Read the model definition and answer for the solid it produces. Units are mm, in the model's axes. Face numbers are marked on the shaded views. A direction names the side the tool comes from. Round coordinates to 2 decimals unless told otherwise and drop trailing zeros. Order: outer loops, then holes, each group sorted by start corner. A loop starts at its lowest first (then second) coordinate and runs counter-clockwise, first axis right, second up. Notation, with made-up numbers: (86, 55) - (139, 55) arc R32 cw to (139, 88) - close; hole circle Ø2 at (-25.75, 53.5). An arc over 180 degrees is marked (long way). Answer as a JSON object with one key per item and string values. Group by question number.
Q1. Consider line 1 (Y direction, x = -30, z = 10.75); line 2 (Y direction, x = -13, z = 13); line 3 (X direction, y = -4.5, z = 13.75). Determine where each line is inside the solid, lowest interval first.
Q2. A cutting plane is placed at C-C on y = -7. Determine the outline of the cut face in (x, z).
Q3. A cutting plane is placed at D-D on x = -17.5. Determine the outline of the cut face in (y, z).
Q4. A tool of negligible diameter and unlimited length cuts with its end or side. For the marked faces 1 and 2, from which of +Z, -Z, +X, -X, +Y, -Y can it reach the whole face along a straight path? Write none if from no direction.
Q5. Given pin 1 Ø2.5 at (x, y) = (-30, 0) entering from +Z; pin 2 Ø3 at (y, z) = (-4, 11) entering from +X, each flat-ended and moving along its own axis, determine where each tip first touches the part or whether it passes through.
Q6. A cutting plane is placed at A-A on x = -30. Determine the outline of the cut face in (y, z).
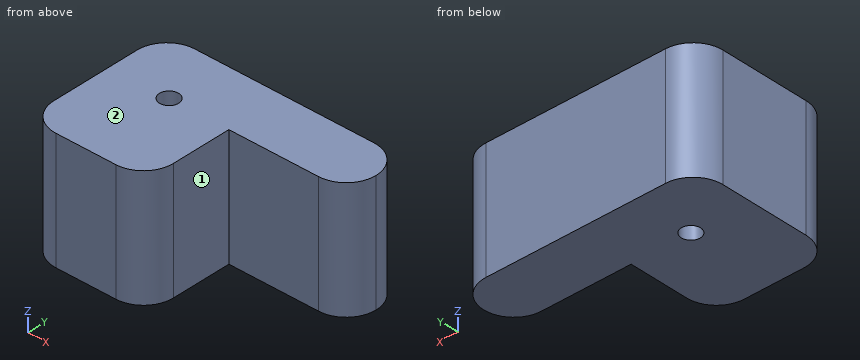
```python
from build123d import *

# Parameters (mm, degrees)
SKETCH_1_W          = 40
SKETCH_1_H          = 10
EXTRUDE_1_DEPTH     = 20
SKETCH_2_W          = 20
SKETCH_2_H          = 25
EXTRUDE_2_DEPTH     = 20
FILLET_1_R          = 5
SKETCH_3_R          = 1.6
CUT_EXTRUDE_1_DEPTH = 48.16990566


with BuildPart() as part:
    # 草图1 → 凸台-拉伸1 (new body)
    with BuildSketch(Plane.XY):
        with Locations((-20, 5)):
            Rectangle(SKETCH_1_W, SKETCH_1_H)
    extrude(amount=EXTRUDE_1_DEPTH)

    # 草图2 → 凸台-拉伸2 (add)
    with BuildSketch(Plane.XY.offset(20)):
        with Locations((-30, -2.5)):
            Rectangle(SKETCH_2_W, SKETCH_2_H)
    extrude(amount=-EXTRUDE_2_DEPTH)

    # 圆角1
    fillet_1_edges = [part.edges().sort_by_distance(p)[0] for p in [
        (0, 10, 10),
        (0, 0, 10),
        (-20, -15, 10),
        (-40, -15, 10),
        (-40, 10, 10),
    ]]
    fillet(fillet_1_edges, radius=FILLET_1_R - 0.0001)  # a hair under: the kernel refuses the full size

    # 草图3 → 切除-拉伸1 (cut, through all)
    with BuildSketch(Plane.XY.offset(20)):
        with Locations((-30, 0)):
            Circle(SKETCH_3_R)
    extrude(amount=-CUT_EXTRUDE_1_DEPTH, mode=Mode.SUBTRACT)


solid = part.part
```
Result set:
{
 "1": {"line 1": "y = -15 to -1.6, 1.6 to 10", "line 2": "y = 0 to 10", "line 3": "x = -40 to -20"},
 "2": {"outline": "(-40, 0) - (-20, 0) - (-20, 20) - (-40, 20) - close"},
 "3": {"outline": "(0, 0) - (10, 0) - (10, 20) - (0, 20) - close"},
 "4": {"face 1": "+Z, -Z, +X, -Y", "face 2": "+Z, +X, -X, +Y, -Y"},
 "5": {"pin 1": "passes through", "pin 2": "stops at x = -20"},
 "6": {"outline": "(-15, 0) - (-1.6, 0) - (-1.6, 20) - (-15, 20) - close; (1.6, 0) - (10, 0) - (10, 20) - (1.6, 20) - close"}
}
